CAD build for the part. Positions are in the model's coordinates, mm. Give positions to 0.01 mm unless a question says otherwise; leave off trailing zeros. Loops run counter-clockwise (first coordinate to the right, second up) from the corner with the lowest first, then second, coordinate; pieces in that order, holes last. Notation, with made-up numbers: (15.5, 41.25) -> (19.5, 41.25) arc R22 cw to (19.5, 77.25) -> close; hole circle Ø5 at (-23, 5.25). An arc over 180 degrees is marked (long way). Use one line per item in the form item = value.
```python
from build123d import *

# Parameters (mm, degrees)
F0_W     = 70
F0_H     = 60
F0_W_2   = 220
F0_H_2   = 50
F1_DEPTH = 3
F2_R     = 2.05
F3_DEPTH = 25
F4_R     = 5


# Not quite as in the source:
# - a feature names something its author has since deleted; it is built from what else it names


with BuildPart() as f1:
    # F0 (on Top) → F1 (new body)
    with BuildSketch(Plane.XY):
        Polygon((35, -15), (110, -15), (110, 15), (-110, 15), (-110, -15), (-35, -15), align=None)
        with Locations((0, -45)):
            Rectangle(F0_W, F0_H)
        with Locations((0, 40)):
            Rectangle(F0_W_2, F0_H_2)
    extrude(amount=F1_DEPTH)

    # F2 (on face) → F3 (cut)
    with BuildSketch(Plane.XY.offset(3)):
        with Locations((-100, 0)):
            Circle(F2_R)
        with Locations((100, 0)):
            Circle(F2_R)
        with BuildLine():
            ThreePointArc((-18.5, 27.5), (-15, 24), (-11.5, 27.5))
            Line((-11.5, 27.5), (-11.5, 38.5))
            ThreePointArc((-11.5, 38.5), (-15, 42), (-18.5, 38.5))
            Line((-18.5, 38.5), (-18.5, 27.5))
        make_face()
        with BuildLine():
            ThreePointArc((11.5, 27.5), (15, 24), (18.5, 27.5))
            Line((18.5, 27.5), (18.5, 38.5))
            ThreePointArc((18.5, 38.5), (15, 42), (11.5, 38.5))
            Line((11.5, 38.5), (11.5, 27.5))
        make_face()
        with BuildLine():
            ThreePointArc((-18.5, -65.5), (-15, -69), (-11.5, -65.5))
            Line((-11.5, -65.5), (-11.5, -54.5))
            ThreePointArc((-11.5, -54.5), (-15, -51), (-18.5, -54.5))
            Line((-18.5, -54.5), (-18.5, -65.5))
        make_face()
        with BuildLine():
            ThreePointArc((11.5, -65.5), (15, -69), (18.5, -65.5))
            Line((18.5, -65.5), (18.5, -54.5))
            ThreePointArc((18.5, -54.5), (15, -51), (11.5, -54.5))
            Line((11.5, -54.5), (11.5, -65.5))
        make_face()
        with Locations((-100, 60)):
            Circle(F2_R)
        with Locations((100, 60)):
            Circle(F2_R)
        with BuildLine():
            ThreePointArc((-18.5, -10.5), (-15, -14), (-11.5, -10.5))
            Line((-11.5, -10.5), (-11.5, 0.5))
            ThreePointArc((-11.5, 0.5), (-15, 4), (-18.5, 0.5))
            Line((-18.5, 0.5), (-18.5, -10.5))
        make_face()
        with BuildLine():
            ThreePointArc((11.5, -10.5), (15, -14), (18.5, -10.5))
            Line((18.5, -10.5), (18.5, 0.5))
            ThreePointArc((18.5, 0.5), (15, 4), (11.5, 0.5))
            Line((11.5, 0.5), (11.5, -10.5))
        make_face()
    extrude(amount=-F3_DEPTH, mode=Mode.SUBTRACT)

    # F4
    f4_edges = [f1.edges().sort_by_distance(p)[0] for p in [
        (-110, -15, 1.5),
        (110, -15, 1.5),
        (110, 65, 1.5),
        (-110, 65, 1.5),
    ]]
    fillet(f4_edges, radius=F4_R)


solid = f1.part
```
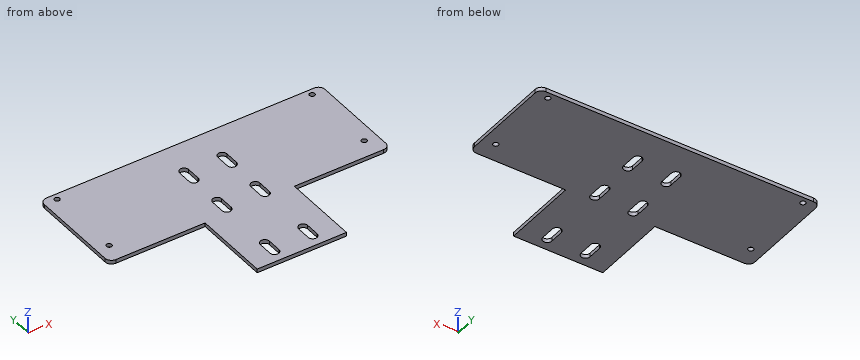
1. Cut at C-C, the plane y = -5.5. Write the cut outline in (x, z).
Result sheet:
outline = (-110, 0) -> (-18.5, 0) -> (-18.5, 3) -> (-110, 3) -> close; (-11.5, 0) -> (11.5, 0) -> (11.5, 3) -> (-11.5, 3) -> close; (18.5, 0) -> (110, 0) -> (110, 3) -> (18.5, 3) -> close
2. Cut at B-B, the plane x = 15. Write the cut outline in (y, z).
Result sheet:
outline = (-75, 0) -> (-69, 0) -> (-69, 3) -> (-75, 3) -> close; (-51, 0) -> (-14, 0) -> (-14, 3) -> (-51, 3) -> close; (4, 0) -> (24, 0) -> (24, 3) -> (4, 3) -> close; (42, 0) -> (65, 0) -> (65, 3) -> (42, 3) -> close
3. Cut at A-A, the plane y = -61.5. Write the cut outline in (x, z), then the cut area to 3 significant figures.
Result sheet:
outline = (-35, 0) -> (-18.5, 0) -> (-18.5, 3) -> (-35, 3) -> close; (-11.5, 0) -> (11.5, 0) -> (11.5, 3) -> (-11.5, 3) -> close; (18.5, 0) -> (35, 0) -> (35, 3) -> (18.5, 3) -> close
area = 168 mm^2
4. Drill centre lines: line 1 (Y direction, x = -100, z = 2.05); line 2 (X direction, y = -52, z = 1.6); line 3 (X direction, y = -39.5, z = 2.15). Where is each one in solid material? Low to high.
Result sheet:
line_1 = -15 to -2.05, 2.05 to 57.95, 62.05 to 65
line_2 = -35 to -17.45, -12.55 to 12.55, 17.45 to 35
line_3 = -35 to 35
5. Drop a flat-ended pin along its axis: P1, Ø0.9, axis at y = -58, z = 2, coming from the -X side. Give the stop position or say it passes through.
Result sheet:
P1 = -35
6. Cut at D-D, the plane z = 1.2. State how many separate pieces and enclosed holes the cut face has, then the cut area to 3 significant figures.
Result sheet:
separate_pieces = 1
enclosed_holes = 10
area = 21,000 mm^2
